```python
from build123d import *

# Parameters (mm, degrees)
SKETCH1_R                        = 39.624
SKETCH1_R_2                      = 38.227
BOSS_EXTRUDE1_DEPTH              = 414.3375
CUT_EXTRUDE1_START               = -1.438371
SKETCH2_R                        = 1.778
CUT_EXTRUDE1_DEPTH               = 1.438371
CIRPATTERN1_COUNT                = 3
PRESSURE_START                   = -1.471239
SKETCH3_R                        = 2.38125
PRESSURE_EQUALIZATION_HOLE_DEPTH = 1.471239
CIRPATTERN2_COUNT                = 3
SKETCH4_R                        = 1.7859375
CUT_EXTRUDE3_DEPTH               = 1.438742
CIRPATTERN3_COUNT                = 3


with BuildPart() as part:
    # Sketch1 → Boss-Extrude1 (new body)
    with BuildSketch(Plane(origin=(0, 0, 0), x_dir=(1, 0, 0), z_dir=(0, 1, 0))):
        Circle(SKETCH1_R)
        Circle(SKETCH1_R_2, mode=Mode.SUBTRACT)
    extrude(amount=BOSS_EXTRUDE1_DEPTH)

    # Sketch2 → Cut-Extrude1 (cut)
    with BuildSketch(Plane(origin=(-19.812, 0, 34.3153906), x_dir=(0, -1, 0), z_dir=(-0.5, 0, 0.866025404)).offset(CUT_EXTRUDE1_START)):
        with Locations((-76.2, 0)):
            Circle(SKETCH2_R)
    cut_extrude1 = extrude(amount=CUT_EXTRUDE1_DEPTH, mode=Mode.SUBTRACT)

    # CirPattern1: Cut-Extrude1 ×3 about axis
    cirpattern1_axis = Axis((0, -7.62, 0), (0, 1, 0))
    for i in range(1, CIRPATTERN1_COUNT):
        add(cut_extrude1.rotate(cirpattern1_axis, i * 360 / CIRPATTERN1_COUNT), mode=Mode.SUBTRACT)

    # Sketch3 → Pressure Equalization Hole (cut)
    with BuildSketch(Plane(origin=(-19.812, 0, 34.3153906), x_dir=(0, -1, 0), z_dir=(-0.5, 0, 0.866025404)).offset(PRESSURE_START)):
        with Locations((-207.16875, 0)):
            Circle(SKETCH3_R)
    pressure_equalization_hole = extrude(amount=PRESSURE_EQUALIZATION_HOLE_DEPTH, mode=Mode.SUBTRACT)

    # CirPattern2: Pressure Equalization Hole ×3 about axis
    cirpattern2_axis = Axis((0, -7.62, 0), (0, 1, 0))
    for i in range(1, CIRPATTERN2_COUNT):
        add(pressure_equalization_hole.rotate(cirpattern2_axis, i * 360 / CIRPATTERN2_COUNT), mode=Mode.SUBTRACT)

    # Sketch4 → Cut-Extrude3 (cut)
    with BuildSketch(Plane(origin=(39.624, 0, 0), x_dir=(0, -1, 0), z_dir=(-1, 0, 0))):
        with Locations((-380.5301, 0)):
            Circle(SKETCH4_R)
    cut_extrude3 = extrude(amount=CUT_EXTRUDE3_DEPTH, mode=Mode.SUBTRACT)

    # CirPattern3: Cut-Extrude3 ×3 about axis
    cirpattern3_axis = Axis((0, -7.62, 0), (0, 1, 0))
    for i in range(1, CIRPATTERN3_COUNT):
        add(cut_extrude3.rotate(cirpattern3_axis, i * 360 / CIRPATTERN3_COUNT), mode=Mode.SUBTRACT)


solid = part.part
```
Could you check a few things on this model? Use its own coordinates, in mm. Round coordinates to 2 decimals unless told otherwise and drop trailing zeros. Loops run counter-clockwise (first coordinate to the right, second up) from the corner with the lowest first, then second, coordinate; pieces in that order, holes last. Notation, with made-up numbers: M 67.25,64 L 85.25,64 A26 cw 85.25,84 Z; hole C 55.25,50.25 d11. An arc over 180 degrees is marked long. Answer as CSV lines item,"result".
1) If I drill on probe 1 along Y at (x, z) = (39, 0); probe 2 along X at (y, z) = (286, 0); probe 3 along X at (y, z) = (41.5, -14), over which ranges is the centre line in solid material (lowest first)?
From the geometry:
probe 1,"0 to 74.42, 77.98 to 204.79, 209.55 to 378.74, 382.32 to 414.34"
probe 2,"-39.62 to -38.23, 38.23 to 39.62"
probe 3,"-37.07 to -35.57, 35.57 to 37.07"
2) Imagine slicing it at A-A on x = 0. List the corners of the cut face in (y, z) for me, and give its area (3 significant figures).
From the geometry:
outline,"M 0,-39.62 L 414.34,-39.62 L 414.34,-38.23 L 0,-38.23 Z; M 0,38.23 L 414.34,38.23 L 414.34,39.62 L 0,39.62 Z"
area,"1,160 mm^2"
3) For pin 1 Ø4 at (y, z) = (332, -26.5) entering from -X; pin 2 Ø4 at (y, z) = (80.5, 20.5) entering from +X; pin 3 Ø3 at (y, z) = (76.2, 0) entering from +X, each with a flat end and sliding along its axis, tell me the tip position at first contact or that it passes through.
From the geometry:
pin 1,"x = -31.14"
pin 2,"x = 35.04"
pin 3,"x = -38.2"
4) We'd pull the mould along X, two halves only. Please class faces 1 (the cylindrical face through (-5.158, 204.268, -39.287)), 2 (the flat face through (-32.5, 0, -20.7)), 3 (the cylindrical face through (-28.17, 204.27, -25.84)): released by +X, released by -X, zero draft, split by the parting line, or undercut.
From the geometry:
face 1,"split by the parting line"
face 2,"zero draft"
face 3,"undercut"
5) Imagine slicing it at B-B on z = 19.5. List the corners of the cut face in (x, y) for me, and give its area (3 significant figures).
From the geometry:
outline,"M -34.49,0 L -32.88,0 L -32.88,414.34 L -34.49,414.34 Z; M 32.88,0 L 34.49,0 L 34.49,414.34 L 32.88,414.34 Z"
area,"1,340 mm^2"
6) Imagine slicing it at C-C on y = 356. List the corners of the cut face in (x, z) for me, and give its area (3 significant figures).
From the geometry:
outline,"C 0,0 d79.25; hole C 0,0 d76.45"
area,"342 mm^2"
